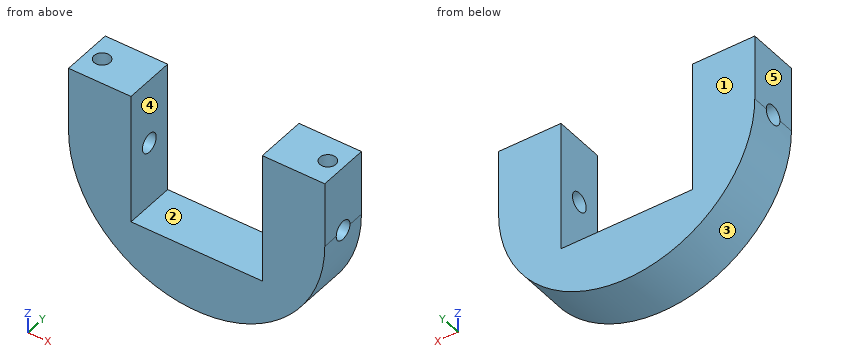
```python
from build123d import *

# Parameters (mm, degrees)
SKETCH1_R                 = 40
BOSS_EXTRUDE1_DEPTH       = 16
SKETCH2_W                 = 41
SKETCH2_H                 = 41
CUT_EXTRUDE1_DEPTH        = 59.787753827
SKETCH13_W                = 61
SKETCH13_H                = 46
BOSS_EXTRUDE4_DEPTH       = 75
SKETCH14_W                = 49
SKETCH14_H                = 67
CUT_EXTRUDE2_DEPTH        = 35
SKETCH15_W                = 49
SKETCH15_H                = 61
CUT_EXTRUDE3_DEPTH        = 5
FILLET1_R                 = 10
FILLET2_R                 = 5
CUT_EXTRUDE5_REACH        = 110.08
SKETCH17_R                = 41
BOSS_EXTRUDE5_DEPTH       = 16
CUT_EXTRUDE4_DEPTH        = 118.224144271
CUT_EXTRUDE4_DEPTH_BACK   = 118.224144271
SKETCH16_R                = 3
F_5_0MM_DOWEL_HOLE1_D     = 5
F_5_0MM_DOWEL_HOLE1_DEPTH = 25
F_5_0MM_DOWEL_HOLE1_TIP   = 1.502151548
CUT_EXTRUDE6_DEPTH        = 109.079831643
CUT_EXTRUDE6_DEPTH_BACK   = 109.079831643
SKETCH21_W                = 80
SKETCH21_H                = 75


with BuildPart() as part:
    # Sketch1 → Boss-Extrude1 (new body)
    with BuildSketch(Plane(origin=(0, 0, 0), x_dir=(1, 0, 0), z_dir=(0, 1, 0))):
        with Locations(Location((0, 0, 0), (0, 0, 270))):
            Circle(SKETCH1_R)
    extrude(amount=BOSS_EXTRUDE1_DEPTH)

    # Sketch2 → Cut-Extrude1 (cut, through all)
    with BuildSketch(Plane(origin=(0, 16, 0), x_dir=(1, 0, 0), z_dir=(0, 1, 0))):
        Rectangle(SKETCH2_W, SKETCH2_H)
    extrude(amount=-CUT_EXTRUDE1_DEPTH, mode=Mode.SUBTRACT)

    # Sketch13 → Boss-Extrude4 (add)
    with BuildSketch(Plane(origin=(0, 0, 20.5), x_dir=(-1, 0, 0), z_dir=(0, 0, -1))):
        with Locations((0, 8)):
            Rectangle(SKETCH13_W, SKETCH13_H)
    extrude(amount=-BOSS_EXTRUDE4_DEPTH)

    # Sketch14 → Cut-Extrude2 (cut)
    with BuildSketch(Plane(origin=(0, 31, 0), x_dir=(1, 0, 0), z_dir=(0, 1, 0))):
        with Locations((0, -62)):
            Rectangle(SKETCH14_W, SKETCH14_H)
    extrude(amount=-CUT_EXTRUDE2_DEPTH, mode=Mode.SUBTRACT)

    # Sketch15 → Cut-Extrude3 (cut)
    with BuildSketch(Plane(origin=(0, -4, 0), x_dir=(1, 0, 0), z_dir=(0, 1, 0))):
        with Locations((0, -59)):
            Rectangle(SKETCH15_W, SKETCH15_H)
    extrude(amount=-CUT_EXTRUDE3_DEPTH, mode=Mode.SUBTRACT)

    # Fillet1
    fillet1_edges = [part.edges().sort_by_distance(p)[0] for p in [
        (-27.5, 31, 95.5),
        (27.5, 31, 95.5),
    ]]
    fillet(fillet1_edges, radius=FILLET1_R)

    # Fillet2
    fillet2_edges = [part.edges().sort_by_distance(p)[0] for p in [
        (0, -9, 89.5),
        (0, -15, 95.5),
        (0, -15, 20.5),
        (0, -9, 28.5),
    ]]
    fillet(fillet2_edges, radius=FILLET2_R - 0.0001)  # a hair under: the kernel refuses the full size

    # Sketch17 → Cut-Extrude5 (cut, up to next)
    with BuildSketch(Plane(origin=(0, 16, 0), x_dir=(1, 0, 0), z_dir=(0, 1, 0)), mode=Mode.PRIVATE) as cut_extrude5_sk1:
        Circle(SKETCH17_R)
    cut_extrude5_tool1 = extrude(cut_extrude5_sk1.sketch, amount=CUT_EXTRUDE5_REACH, mode=Mode.PRIVATE) & part.part
    add(cut_extrude5_tool1.solids().sort_by_distance((0, 16, 0))[0], mode=Mode.SUBTRACT)

    # Sketch18 → Boss-Extrude5 (add)
    with BuildSketch(Plane(origin=(0, 16, 0), x_dir=(1, 0, 0), z_dir=(0, 1, 0))):
        Polygon((20.5, 0), (20.5, -20.5), (-20.5, -20.5), (-20.5, 0), (-40, 0), (-40, -32.874762357), (-24.5, -32.874762357), (-24.5, -28.5), (24.5, -28.5), (24.5, -32.874762357), (40, -32.874762357), (40, 0), align=None)
    extrude(amount=-BOSS_EXTRUDE5_DEPTH)

    # Sketch16 → Cut-Extrude4 (cut, two sides: drawn at the far end of the back side and taken through both)
    with BuildSketch(Plane.ZY.offset(-20.5).offset(-CUT_EXTRUDE4_DEPTH_BACK)):
        with Locations(Location((0, 8, 0), (0, 0, 270))):
            Circle(SKETCH16_R)
    extrude(amount=CUT_EXTRUDE4_DEPTH + CUT_EXTRUDE4_DEPTH_BACK, mode=Mode.SUBTRACT)

    # Ø5.0mm Dowel Hole1
    with Locations(Plane(origin=(-35.25, 8, 32.874762357), x_dir=(1, 0, 0), z_dir=(0, 0, 1))):
        with Locations((0, 0), (70.5, 0)):
            Hole(F_5_0MM_DOWEL_HOLE1_D / 2, depth=F_5_0MM_DOWEL_HOLE1_DEPTH)
            with Locations((0, 0, -(F_5_0MM_DOWEL_HOLE1_DEPTH + F_5_0MM_DOWEL_HOLE1_TIP / 2))):  # 118° drill point
                Cone(0, F_5_0MM_DOWEL_HOLE1_D / 2, F_5_0MM_DOWEL_HOLE1_TIP, mode=Mode.SUBTRACT)

    # Sketch21 → Cut-Extrude6 (cut, two sides: drawn at the far end of the back side and taken through both)
    with BuildSketch(Plane(origin=(0, 16, 0), x_dir=(1, 0, 0), z_dir=(0, 1, 0)).offset(-CUT_EXTRUDE6_DEPTH_BACK)):
        with Locations((0, -58)):
            Rectangle(SKETCH21_W, SKETCH21_H)
    extrude(amount=CUT_EXTRUDE6_DEPTH + CUT_EXTRUDE6_DEPTH_BACK, mode=Mode.SUBTRACT)


solid = part.part
```
The model under review builds one solid part; all positions refer to its coordinate system, in mm. Face numbers are marked on the shaded views. A direction names the side the tool comes from. Round coordinates to 2 decimals unless told otherwise and drop trailing zeros. Loops run counter-clockwise (first coordinate to the right, second up) from the corner with the lowest first, then second, coordinate; pieces in that order, holes last. Notation, with made-up numbers: M 83.5,-9.5 L 100.5,-9.5 A18 cw 100.5,2.5 Z; hole C 74,30 d4. An arc over 180 degrees is marked long. Write item = value, one per line.
Item 1: Machinability: for the marked faces 4 and 5, which of the approach directions +Z, -Z, +X, -X, +Y, -Y give a long, thin tool a straight path to every point of the face, cutting with its end or side? Answer none if there is none.
Return value:
face_4 = +Z, +Y, -Y
face_5 = +Z, -Z, -X, +Y, -Y
Item 2: The part is to be moulded in two halves that separate along X. For the marked faces 1, 2 and 3, say which applies: released by +X, released by -X, zero draft, split by the parting line, or undercut.
Return value:
face_1 = zero draft
face_2 = undercut
face_3 = split by the parting line
Item 3: Take a section at A-A on z = 16. Write out the cut boundary in (x, y), then the cut area to 3 significant figures.
Return value:
outline = M -40,0 L -20.5,0 L -20.5,16 L -40,16 Z; M 20.5,0 L 40,0 L 40,16 L 20.5,16 Z; hole C -35.25,8 d5; hole C 35.25,8 d5
area = 585 mm2
Item 4: Take a section at D-D on z = -7. Write out the cut boundary in (x, y), then the cut area to 3 significant figures.
Return value:
outline = M -39.38,0 L -20.5,0 L -20.5,16 L -39.38,16 Z; M 20.5,0 L 39.38,0 L 39.38,16 L 20.5,16 Z
area = 604 mm2
Item 5: Take a section at C-C on y = 14. Write out the cut boundary in (x, z).
Return value:
outline = M -40,0 A40 ccw 40,0 L 40,20.5 L 20.5,20.5 L 20.5,-20.5 L -20.5,-20.5 L -20.5,20.5 L -40,20.5 Z
Item 6: Insertion check: P1, Ø3, axis at x = 12.5, y = 5.5, coming from the -Z side; P2, Ø7, axis at y = 8, z = 0, coming from the +X side; P3, Ø3, axis at x = 35.25, y = 8, coming from the -Z side; P4, Ø6, axis at x = 20, y = 12.5, coming from the -Z side. Each pin has a flat end and moves straight along its axis. Give the tip position at first contact, or say it passes through.
Return value:
P1 = -38.46
P2 = 40
P3 = -21.47
P4 = -36.21
Item 7: Take a section at B-B on x = 22. Write out the cut boundary in (y, z), then the cut area to 3 significant figures.
Return value:
outline = M 0,-33.41 L 16,-33.41 L 16,20.5 L 0,20.5 Z; hole C 8,0 d6
area = 834 mm2
Item 8: For line 1 (X direction, y = 8, z = 17.5); line 2 (X direction, y = 10.75, z = 16.5); line 3 (Y direction, x = -35.25, z = 11.5), list the stretches that pass through material, from the lowest coordinate up. Write a range as [from, to].
Return value:
line_1 = [-40, -37.75], [-32.75, -20.5], [20.5, 32.75], [37.75, 40]
line_2 = [-40, -20.5], [20.5, 40]
line_3 = [0, 5.5], [10.5, 16]
